```python
from build123d import *

# Parameters (mm, degrees)
SKETCH1_R           = 2.25
BOSS_EXTRUDE1_DEPTH = 25
BOSS_EXTRUDE2_DEPTH = 4


with BuildPart() as part:
    # Sketch1 → Boss-Extrude1 (new body)
    with BuildSketch(Plane(origin=(0, 0, 0), x_dir=(1, 0, 0), z_dir=(0, 1, 0))):
        with Locations(Location((0, 0, 0), (0, 0, 270))):
            Circle(SKETCH1_R)
    extrude(amount=BOSS_EXTRUDE1_DEPTH)

    # Sketch2 → Boss-Extrude2 (add)
    with BuildSketch(Plane(origin=(0, 25, 0), x_dir=(1, 0, 0), z_dir=(0, 1, 0))):
        Polygon((-3.25, -1.876388375), (0, -3.75277675), (3.25, -1.876388375), (3.25, 1.876388375), (0, 3.75277675), (-3.25, 1.876388375), align=None)
    extrude(amount=BOSS_EXTRUDE2_DEPTH)

    # Sketch4 → Cut-Revolve1 (revolve, cut)
    with BuildSketch(Plane(origin=(0, 0, 0), x_dir=(0, 0, -1), z_dir=(1, 0, 0))):
        Polygon((3.25277675, 29), (3.75277675, 28.5), (3.75277675, 29), align=None)
    revolve(axis=Axis((0, 0, 0), (0, 1, 0)), mode=Mode.SUBTRACT)


solid = part.part
```
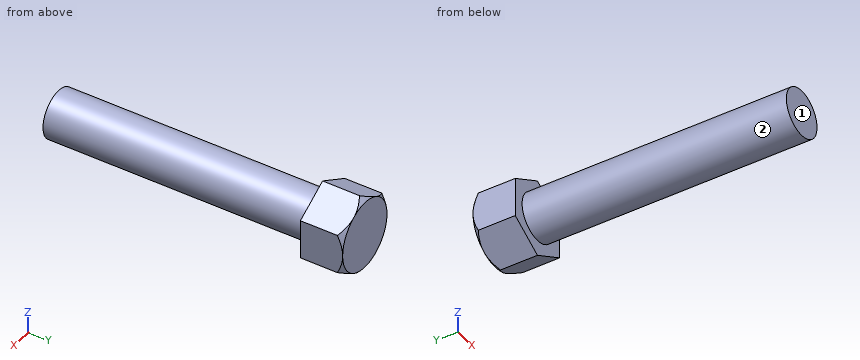
Build history of the part. All positions in model axes, mm. Face numbers are marked on the shaded views. A direction names the side the tool comes from. Round coordinates to 2 decimals unless told otherwise and drop trailing zeros. Write each loop counter-clockwise with the first axis right and the second up, starting at its lowest first coordinate (ties: lowest second). Pieces come first, ordered by that corner, then holes.
1) Drill centre lines: probe 1 along X at (y, z) = (15.5, -1.25); probe 2 along Y at (x, z) = (-1.25, 2); probe 3 along X at (y, z) = (6.75, -1.75). Where is each one in solid material? Low to high.
2) Pin check, flat tip, straight feed: pin 1 (2 mm diameter, centred on x = 0, y = 20.5, fed in from +Z). Stop position of the tip, or through.
3) Band-saw the part on A-A, the plane y = 12.75. List the corners of the cut face in (x, z).
4) 3-axis set-ups, long thin cutter, end or side, ignore diameter. For the marked faces 1 and 2: which of +Z, -Z, +X, -X, +Y, -Y reach the whole face in a straight line?
Ans:
1. probe 1: x = -1.87 to 1.87
1. probe 2: y = 25 to 29
1. probe 3: x = -1.41 to 1.41
2. pin 1: stops at z = 2.25
3. outline: circle Ø4.5 at (0, 0)
4. face 1: +Z, -Z, +X, -X, -Y
4. face 2: -Y
